Source: CAD feature listing. Evaluate the final solid. Frame: model axes, mm. Round coordinates to 2 decimals unless told otherwise and drop trailing zeros. Loops run counter-clockwise (first coordinate to the right, second up) from the corner with the lowest first, then second, coordinate; pieces in that order, holes last.
(1) Section B-B, the plane z = 0.8. Count the separate pieces of the cut face and the enclosed holes in it, plus the area to 3 significant figures.
(2) Material intervals for probe 1 along Y at (x, z) = (9.5, 0.6); probe 2 along X at (y, z) = (-147, 0.9); probe 3 along Z at (x, y) = (25, -50), sorted ascending.
(3) Section A-A, the plane y = -142. Return the cut outline in (x, z).
(4) First-contact query: pin 1 Ø1.8 at (x, z) = (-2.5, 1) entering from +Y; pin 2 Ø8 at (x, y) = (14, -60.5) entering from -Z; pin 3 Ø1.1 at (x, z) = (29.5, 2.5) entering from -Y; pin 4 Ø2.5 at (x, y) = (-0.99, -122.21) entering from +Z. Flat tips, straight axial feed; report the tip coordinate or a pass-through.
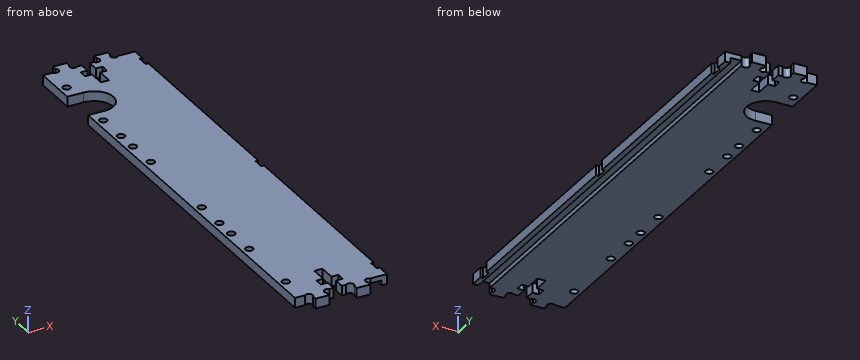
Autodesk Inventor part; units mm, degrees
ref_plane "YZ Plane" through (0, 0, 0) normal (1, 0, 0) x (0, 1, 0)
ref_plane "XZ Plane" through (0, 0, 0) normal (0, 1, 0) x (-1, 0, 0)
ref_plane "XY Plane" through (0, 0, 0) normal (0, 0, 1) x (1, 0, 0)
ref_plane "Work Plane1" through (0, 0, 0) normal (0, 0, 1) x (1, 0, 0)
sketch "Sketch1" plane through (0, 0, 0) normal (0, 0, 1) x (1, 0, 0)
  line L0 (30, 0) -> (23.9528, 0)
  line L1 (30, 0) -> (30, -5)
  line L2 (23.9799, -170) -> (30, -170)
  line L3 (22, -171.9799) -> (22, -173.6)
  line L4 (22, -173.6) -> (17, -173.6)
  line L5 (17, -173.6) -> (17, -171.9799)
  line L6 (15.0201, -170) -> (13.5, -170)
  line L7 (13.5, -170) -> (13.5, -166)
  line L8 (13.5, -166) -> (16, -166)
  line L9 (16, -166) -> (16, -163)
  line L10 (16, -163) -> (13.5, -163)
  line L11 (13.5, -163) -> (13.5, -157)
  line L12 (13.5, -157) -> (10.5, -157)
  line L13 (10.5, -157) -> (10.5, -163)
  line L14 (10.5, -163) -> (8, -163)
  line L15 (8, -163) -> (8, -166)
  line L16 (8, -166) -> (10.5, -166)
  line L17 (10.5, -166) -> (10.5, -170)
  line L18 (10.5, -170) -> (8.9799, -170)
  line L19 (7, -171.9799) -> (7, -173.6)
  line L20 (7, -173.6) -> (2, -173.6)
  line L21 (2, -173.6) -> (2, -171.9799)
  line L22 (0.0201, -170) -> (-3.6, -170)
  line L23 (-3.6, -170) -> (-3.6, 0)
  line L24 (-3.6, 0) -> (0.0472, 0)
  line L25 (2, 1.9528) -> (2, 3.6)
  line L26 (2, 3.6) -> (7, 3.6)
  line L27 (7, 3.6) -> (7, 1.9799)
  line L28 (8.9799, 0) -> (10.5, 0)
  line L29 (10.5, 0) -> (10.5, -4)
  line L30 (10.5, -4) -> (8, -4)
  line L31 (8, -4) -> (8, -7)
  line L32 (8, -7) -> (10.5, -7)
  line L33 (10.5, -7) -> (10.5, -13)
  line L34 (10.5, -13) -> (13.5, -13)
  line L35 (13.5, -13) -> (13.5, -7)
  line L36 (13.5, -7) -> (16, -7)
  line L37 (16, -7) -> (16, -4)
  line L38 (16, -4) -> (13.5, -4)
  line L39 (13.5, -4) -> (13.5, 0)
  line L40 (13.5, 0) -> (15.0472, 0)
  line L41 (17, 1.9528) -> (17, 3.6)
  line L42 (17, 3.6) -> (22, 3.6)
  line L43 (22, 3.6) -> (22, 1.9528)
  line L44 (29, -165) -> (30, -165)
  line L45 (30, -5) -> (29, -5)
  line L46 (29, -5) -> (29, -9)
  line L47 (29, -9) -> (30, -9)
  line L48 (30, -9) -> (30, -83)
  line L49 (30, -83) -> (29, -83)
  line L50 (29, -83) -> (29, -87)
  line L51 (29, -87) -> (30, -87)
  line L52 (30, -87) -> (30, -161)
  line L53 (30, -161) -> (29, -161)
  line L54 (29, -161) -> (29, -165)
  arc A0 (17, -171.9799) -> (15.0201, -170) centre (16.0101, -170.9899) ccw
  arc A1 (8.9799, -170) -> (7, -171.9799) centre (7.9899, -170.9899) ccw
  arc A2 (2, -171.9799) -> (0.0201, -170) centre (1.0101, -170.9899) ccw
  arc A3 (0.0472, 0) -> (2, 1.9528) centre (1.1868, 0.8132) ccw
  arc A4 (7, 1.9799) -> (8.9799, 0) centre (7.9899, 0.9899) ccw
  arc A5 (15.0472, 0) -> (17, 1.9528) centre (16.1868, 0.8132) ccw
  arc A6 (22, 1.9528) -> (23.9528, 0) centre (22.8132, 0.8132) ccw
  line L55 (30, -165) -> (30, -170)
  arc A7 (23.9799, -170) -> (22, -171.9799) centre (22.9899, -170.9899) ccw
  circle A8 centre (-0.9899, -159.0101) radius 1.4
  circle A9 centre (-0.8132, -134.0132) radius 1.4
  circle A10 centre (-0.9899, -122.2101) radius 1.4
  circle A11 centre (-0.9899, -114.1899) radius 1.4
  circle A12 centre (-0.9899, -102.2101) radius 1.4
  circle A13 centre (-0.8132, -67.6132) radius 1.4
  circle A14 centre (-0.9899, -55.8101) radius 1.4
  circle A15 centre (-0.9899, -47.7899) radius 1.4
  circle A16 centre (-0.9899, -35.8101) radius 1.4
  circle A17 centre (-0.8132, -10.8132) radius 1.4
  point P0 (0, 0)
  point P1 (22, 0)
  point P2 (22, -170)
  point P3 (17, -170)
  point P4 (7, -170)
  point P5 (2, -170)
  point P6 (0, -160)
  point P7 (0, -123.2)
  point P8 (0, -113.2)
  point P9 (0, -103.2)
  point P10 (0, -56.8)
  point P11 (0, -46.8)
  point P12 (0, -36.8)
  point P13 (2, 0)
  point P14 (7, 0)
  point P15 (17, 0)
  point P16 (-1.9799, -160)
  point P17 (-1.9528, -133.2)
  point P18 (-1.9799, -123.2)
  point P19 (-1.9799, -113.2)
  point P20 (-1.9799, -103.2)
  point P21 (-1.9528, -66.8)
  point P22 (-1.9799, -56.8)
  point P23 (-1.9799, -46.8)
  point P24 (-1.9799, -36.8)
  point P25 (-1.9528, -10)
  point P26 (0, -34.8201)
  point P27 (0, -11.9528)
  point P28 (0, -54.8201)
  point P29 (0, -48.7799)
  point P30 (0, -101.2201)
  point P31 (0, -68.7528)
  point P32 (0, -121.2201)
  point P33 (0, -115.1799)
  point P34 (0, -158.0201)
  point P35 (0, -135.1528)
extrude "Extrusion1" add sketch "Sketch1" along normal blind 3.6
sketch "Sketch3" plane through (0, 0, 0) normal (0, 0, -1) x (-1, 0, 0)
  line L0 (-28, -170) -> (-24, -170)
  line L1 (-28, 0) -> (-28, -170)
  line L2 (-24, 0) -> (-28, 0)
  line L3 (-24, 0) -> (-24, -170)
  point P0 (0, 0)
extrude "Extrusion3" cut sketch "Sketch3" against normal blind 1.8
sketch "Sketch16" plane through (0, 0, 3.6) normal (0, 0, 1) x (1, 0, 0)
  line L0 (30, -87) -> (29, -87)
  line L1 (29, -87) -> (29, -83)
  line L2 (29, -83) -> (30, -83)
  line L3 (30, -83) -> (30, -9)
  line L4 (30, -9) -> (29, -9)
  line L5 (29, -9) -> (29, -5)
  line L6 (29, -5) -> (30, -5)
  line L7 (30, -5) -> (30, 0)
  line L8 (30, 0) -> (23.9528, 0)
  arc A0 (22, 1.9528) -> (23.9528, 0) centre (22.8132, 0.8132) ccw
  line L9 (22, 1.9528) -> (22, 3.6)
  line L10 (22, 3.6) -> (17, 3.6)
  line L11 (17, 3.6) -> (17, 1.9528)
  arc A1 (15.0472, 0) -> (17, 1.9528) centre (16.1868, 0.8132) ccw
  line L12 (15.0472, 0) -> (13.5, 0)
  line L13 (13.5, 0) -> (13.5, -4)
  line L14 (13.5, -4) -> (16, -4)
  line L15 (16, -4) -> (16, -7)
  line L16 (16, -7) -> (13.5, -7)
  line L17 (13.5, -7) -> (13.5, -13)
  line L18 (13.5, -13) -> (10.5, -13)
  line L19 (10.5, -13) -> (10.5, -7)
  line L20 (10.5, -7) -> (8, -7)
  line L21 (8, -7) -> (8, -4)
  line L22 (8, -4) -> (10.5, -4)
  line L23 (10.5, -4) -> (10.5, 0)
  line L24 (10.5, 0) -> (8.9799, 0)
  arc A2 (7, 1.9799) -> (8.9799, 0) centre (7.9899, 0.9899) ccw
  line L25 (7, 1.9799) -> (7, 3.6)
  line L26 (7, 3.6) -> (2, 3.6)
  line L27 (2, 3.6) -> (2, 1.9528)
  arc A3 (0.0472, 0) -> (2, 1.9528) centre (1.1868, 0.8132) ccw
  line L28 (0.0472, 0) -> (-3.6, 0)
  circle A4 centre (-0.8132, -10.8132) radius 1.4
  circle A5 centre (-0.9899, -35.8101) radius 1.4
  circle A6 centre (-0.9899, -47.7899) radius 1.4
  circle A7 centre (-0.9899, -55.8101) radius 1.4
  circle A8 centre (-0.8132, -67.6132) radius 1.4
  circle A9 centre (-0.9899, -102.2101) radius 1.4
  circle A10 centre (-0.9899, -114.1899) radius 1.4
  circle A11 centre (-0.9899, -122.2101) radius 1.4
  circle A12 centre (-0.8132, -134.0132) radius 1.4
  circle A13 centre (-0.9899, -159.0101) radius 1.4
  line L29 (-3.6, 0) -> (-3.6, -170)
  line L30 (-3.6, -170) -> (0.0201, -170)
  arc A14 (2, -171.9799) -> (0.0201, -170) centre (1.0101, -170.9899) ccw
  line L31 (2, -171.9799) -> (2, -173.6)
  line L32 (2, -173.6) -> (7, -173.6)
  line L33 (7, -173.6) -> (7, -171.9799)
  arc A15 (8.9799, -170) -> (7, -171.9799) centre (7.9899, -170.9899) ccw
  line L34 (8.9799, -170) -> (10.5, -170)
  line L35 (10.5, -170) -> (10.5, -166)
  line L36 (10.5, -166) -> (8, -166)
  line L37 (8, -166) -> (8, -163)
  line L38 (8, -163) -> (10.5, -163)
  line L39 (10.5, -163) -> (10.5, -157)
  line L40 (10.5, -157) -> (13.5, -157)
  line L41 (13.5, -157) -> (13.5, -163)
  line L42 (13.5, -163) -> (16, -163)
  line L43 (16, -163) -> (16, -166)
  line L44 (16, -166) -> (13.5, -166)
  line L45 (13.5, -166) -> (13.5, -170)
  line L46 (13.5, -170) -> (15.0201, -170)
  arc A16 (17, -171.9799) -> (15.0201, -170) centre (16.0101, -170.9899) ccw
  line L47 (17, -171.9799) -> (17, -173.6)
  line L48 (17, -173.6) -> (22, -173.6)
  line L49 (22, -173.6) -> (22, -171.9799)
  arc A17 (23.9799, -170) -> (22, -171.9799) centre (22.9899, -170.9899) ccw
  line L50 (23.9799, -170) -> (30, -170)
  line L51 (30, -170) -> (30, -165)
  line L52 (30, -165) -> (29, -165)
  line L53 (29, -165) -> (29, -161)
  line L54 (29, -161) -> (30, -161)
  line L55 (30, -161) -> (30, -87)
  line L56 (0, -30.4) -> (-3.6, -30.4)
  line L57 (0, -16.4) -> (-3.6, -16.4)
  line L58 (-3.6, -23.3865) -> (2.4, -23.3865) construction
  line L59 (-3.6, -16.3729) -> (2.4, -16.3729)
  line L60 (2.4, -30.4) -> (-3.6, -30.4)
  arc A18 (-3.6, -16.3729) -> (-3.6, -30.4) centre (-3.6, -23.3865) ccw
  arc A19 (2.4, -30.4) -> (2.4, -16.3729) centre (2.4, -23.3865) ccw
  point P0 (0, 0)
  point P1 (-0.6, -23.3865)
  dimension "d39" = 6
extrude "Extrusion6" cut sketch "Sketch16" against normal through all contours A18 L29 | L29 L59 A19 L60 L56
sketch "Sketch17" plane through (0, 0, 3.6) normal (0, 0, 1) x (1, 0, 0)
  line L0 (-3.6, -16.3729) -> (2.4, -16.3729)
  arc A0 (2.4, -30.4) -> (2.4, -16.3729) centre (2.4, -23.3865) ccw
  line L1 (2.4, -30.4) -> (-3.6, -30.4)
  circle A1 centre (-0.9899, -35.8101) radius 1.4
  circle A2 centre (-0.9899, -47.7899) radius 1.4
  circle A3 centre (-0.9899, -55.8101) radius 1.4
  circle A4 centre (-0.8132, -67.6132) radius 1.4
  circle A5 centre (-0.9899, -102.2101) radius 1.4
  circle A6 centre (-0.9899, -114.1899) radius 1.4
  circle A7 centre (-0.9899, -122.2101) radius 1.4
  circle A8 centre (-0.8132, -134.0132) radius 1.4
  circle A9 centre (-0.9899, -159.0101) radius 1.4
  line L2 (-3.6, 0) -> (-3.6, -16.3729)
  line L3 (-3.6, -170) -> (0.0201, -170)
  arc A10 (2, -171.9799) -> (0.0201, -170) centre (1.0101, -170.9899) ccw
  line L4 (2, -171.9799) -> (2, -173.6)
  line L5 (2, -173.6) -> (7, -173.6)
  line L6 (7, -173.6) -> (7, -171.9799)
  arc A11 (8.9799, -170) -> (7, -171.9799) centre (7.9899, -170.9899) ccw
  line L7 (8.9799, -170) -> (10.5, -170)
  line L8 (10.5, -170) -> (10.5, -166)
  line L9 (10.5, -166) -> (8, -166)
  line L10 (8, -166) -> (8, -163)
  line L11 (8, -163) -> (10.5, -163)
  line L12 (10.5, -163) -> (10.5, -157)
  line L13 (10.5, -157) -> (13.5, -157)
  line L14 (13.5, -157) -> (13.5, -163)
  line L15 (13.5, -163) -> (16, -163)
  line L16 (16, -163) -> (16, -166)
  line L17 (16, -166) -> (13.5, -166)
  line L18 (13.5, -166) -> (13.5, -170)
  line L19 (13.5, -170) -> (15.0201, -170)
  arc A12 (17, -171.9799) -> (15.0201, -170) centre (16.0101, -170.9899) ccw
  line L20 (17, -171.9799) -> (17, -173.6)
  line L21 (17, -173.6) -> (22, -173.6)
  line L22 (22, -173.6) -> (22, -171.9799)
  arc A13 (23.9799, -170) -> (22, -171.9799) centre (22.9899, -170.9899) ccw
  line L23 (23.9799, -170) -> (30, -170)
  line L24 (30, -170) -> (30, -165)
  line L25 (30, -165) -> (29, -165)
  line L26 (29, -165) -> (29, -161)
  line L27 (29, -161) -> (30, -161)
  line L28 (30, -161) -> (30, -87)
  line L29 (30, -87) -> (29, -87)
  line L30 (29, -87) -> (29, -83)
  line L31 (29, -83) -> (30, -83)
  line L32 (30, -83) -> (30, -9)
  line L33 (30, -9) -> (29, -9)
  line L34 (29, -9) -> (29, -5)
  line L35 (29, -5) -> (30, -5)
  line L36 (30, -5) -> (30, 0)
  line L37 (30, 0) -> (23.9528, 0)
  arc A14 (22, 1.9528) -> (23.9528, 0) centre (22.8132, 0.8132) ccw
  line L38 (22, 1.9528) -> (22, 3.6)
  line L39 (22, 3.6) -> (17, 3.6)
  line L40 (17, 3.6) -> (17, 1.9528)
  arc A15 (15.0472, 0) -> (17, 1.9528) centre (16.1868, 0.8132) ccw
  line L41 (15.0472, 0) -> (13.5, 0)
  line L42 (13.5, 0) -> (13.5, -4)
  line L43 (13.5, -4) -> (16, -4)
  line L44 (16, -4) -> (16, -7)
  line L45 (16, -7) -> (13.5, -7)
  line L46 (13.5, -7) -> (13.5, -13)
  line L47 (13.5, -13) -> (10.5, -13)
  line L48 (10.5, -13) -> (10.5, -7)
  line L49 (10.5, -7) -> (8, -7)
  line L50 (8, -7) -> (8, -4)
  line L51 (8, -4) -> (10.5, -4)
  line L52 (10.5, -4) -> (10.5, 0)
  line L53 (10.5, 0) -> (8.9799, 0)
  arc A16 (7, 1.9799) -> (8.9799, 0) centre (7.9899, 0.9899) ccw
  line L54 (7, 1.9799) -> (7, 3.6)
  line L55 (7, 3.6) -> (2, 3.6)
  line L56 (2, 3.6) -> (2, 1.9528)
  arc A17 (0.0472, 0) -> (2, 1.9528) centre (1.1868, 0.8132) ccw
  line L57 (0.0472, 0) -> (-3.6, 0)
  circle A18 centre (-0.8132, -10.8132) radius 1.4
  line L58 (0, -153.6) -> (-3.6, -153.6)
  line L59 (0, -135.1528) -> (0, -158.0201)
  arc A19 (-0.2318, -139.5767) -> (5.2144, -151.2768) centre (0, -146.5865) ccw
  arc A20 (8.7055, -149.9855) -> (3.0039, -137.7368) centre (9.7399, -142.0526) ccw
  arc A21 (-0.2318, -139.5767) -> (3.0039, -137.7368) centre (-0.3641, -135.5789) ccw
  arc A22 (8.7055, -149.9855) -> (5.2144, -151.2768) centre (8.1883, -153.9519) ccw
  line L60 (-3.6, -30.4) -> (-3.6, -170)
  point P0 (0, 0)
  dimension "d42" = 16
  dimension "d43" = 4
extrude "Extrusion7" [suppressed]
equation "\"d0\" = wood_thickness"
equation "\"d7\" = deep_for_sliding_cover"
properties part number "side_top"
Output values:
1. separate pieces: 2
1. enclosed holes: 10
1. area: 4,750 mm2
2. probe 1: y = -170 to -166, -163 to -7, -4 to 0
2. probe 2: x = -3.6 to 24, 28 to 30
2. probe 3: z = 1.8 to 3.6
3. outline: (-3.6, 0) - (24, 0) - (24, 1.8) - (28, 1.8) - (28, 0) - (30, 0) - (30, 3.6) - (-3.6, 3.6) - close
4. pin 1: stops at y = 0
4. pin 2: stops at z = 0
4. pin 3: stops at y = -170
4. pin 4: passes through
